from build123d import *

# Parameters (mm, degrees)
SKETCH1_R           = 12.7
BOSS_EXTRUDE1_DEPTH = 7.62


with BuildPart() as part:
    # Sketch1 → Boss-Extrude1 (new body)
    with BuildSketch(Plane(origin=(0, 0, 0), x_dir=(1, 0, 0), z_dir=(0, 1, 0))):
        with BuildLine():
            Line((-14.199031657, 12.7), (-101.6, 12.7))
            add(Edge.make_bspline(
                [(-101.6, 12.7), (-184.883349987, 44.014741237), (-269.184277242, 0)],
                knots=[0, 0, 0, 1, 1, 1], degree=2))
            add(Edge.make_bspline(
                [(-101.6, -12.7), (-184.883349987, -44.014741237), (-269.184277242, 0)],
                knots=[0, 0, 0, 1, 1, 1], degree=2))
            Line((-101.6, -12.7), (-14.199031657, -12.7))
            ThreePointArc((-14.199031657, -12.7), (19.05, 0), (-14.199031657, 12.7))
        make_face()
        with Locations(Location((0, 0, 0), (0, 0, 90))):
            Circle(SKETCH1_R, mode=Mode.SUBTRACT)
    extrude(amount=BOSS_EXTRUDE1_DEPTH)


solid = part.part
Could you check a few things on this model? Use its own coordinates, in mm. A direction names the side the tool comes from. Give positions to 0.01 mm unless a question says otherwise; leave off trailing zeros. Order: outer loops, then holes, each group sorted by start corner. A loop starts at its lowest first (then second) coordinate and runs counter-clockwise, first axis right, second up. Notation, with made-up numbers: (11, -21) - (37, -21) arc R24 cw to (37, -8) - close; hole circle Ø8 at (5.25, 9.5). An arc over 180 degrees is marked (long way). Return JSON: item names as keys, results as strings. Group by question number.
Q1. Please list where these lines run through material, in increasing order: line 1 along X through (y, z) = (5.75, 0); line 2 along Z through (x, y) = (-59.5, 3.75); line 3 along X through (y, z) = (4, 1). Write a range as [from, to].
Q2. Suppose I cut it at B-B, the plane x = -36.5. Please give me the cut outline in (y, z), and give its area (3 significant figures).
Q3. Suppose I cut it at A-A, the plane x = 0. Please give me the cut outline in (y, z).
Q4. Will these pins go through, and if not, where does the flat tip stop? pin 1 Ø15 at (x, z) = (0, 0) entering from +Y; pin 2 Ø2 at (y, z) = (1.5, 1.5) entering from -X; pin 3 Ø3 at (x, y) = (-16.5, 3) entering from -Z.
Q5. Thinking about a two-plate mould opening in X: for faces 1 (the face through (-136, 0, -3)), 2 (the face through (7.7, 3.8, 10.1)), which applies, pulls with the +X half, pulls with the -X half, needs draft (parallel to the pull), parting line crosses it, or undercut?
Q6. Which directions (+Z, -Z, +X, -X, +Y, -Y) give clear straight access to the entire face, cutting with the end or side of a thin tool? Please do faces 3 (the face through (19.04, 3.76, 0.64)), 4 (the face through (-59, 4, 12.7)), 5 (the face through (-57, 4, -12.7)).
Resolved:
{
 "1": {"line 1": "x = [-269.18, -12.7], [12.7, 19.05]", "line 2": "z = [-12.7, 12.7]", "line 3": "x = [-267.25, -12.66], [12.66, 19.02]"},
 "2": {"outline": "(0, -12.7) - (7.62, -12.7) - (7.62, 12.7) - (0, 12.7) - close", "area": "194 mm2"},
 "3": {"outline": "(0, -19.05) - (7.62, -19.05) - (7.62, -12.7) - (0, -12.7) - close; (0, 12.7) - (7.62, 12.7) - (7.62, 19.05) - (0, 19.05) - close"},
 "4": {"pin 1": "passes through", "pin 2": "stops at x = -268.22", "pin 3": "stops at z = -12.7"},
 "5": {"face 1": "needs draft", "face 2": "undercut"},
 "6": {"face 3": "+Y, -Y", "face 4": "+Z, +Y, -Y", "face 5": "-Z, +Y, -Y"}
}
